Build history of the part. All positions in model axes, mm. A direction names the side the tool comes from. Give positions to 0.01 mm unless a question says otherwise; leave off trailing zeros. Loops run counter-clockwise (first coordinate to the right, second up) from the corner with the lowest first, then second, coordinate; pieces in that order, holes last. Notation, with made-up numbers: (44, -23.75) -> (75, -23.75) arc R15 ccw to (75, 0.25) -> close; hole circle Ø7 at (30, 8). An arc over 180 degrees is marked (long way). One line per question, with ' | ' between items. Start each with the question number.
(1) Slice it at C-C, the plane x = 30. Write the cut outline in (y, z).
(2) Drill centre lines: L1, parallel to X at y = 66.5, z = 31.5; L2, parallel to Y at x = 49, z = 38.5; L3, parallel to Z at x = 30, y = 0.8. Where is each one in solid material? Low to high. Write a range as from..to.
(3) Slice it at B-B, the plane z = 30. Write the cut outline in (x, y), then the cut area to 3 significant figures.
(4) Mould opens along X. For faces 1 (the face through (29.479, 1.014, 26.034)), 2 (the face through (108.99, 2.85, 29.58)), 3 (the face through (50, 0, 30)) say: pulls with the +X half, pulls with the -X half, needs draft (parallel to the pull), parting line crosses it, or undercut.
(5) 3-axis set-ups, long thin cutter, end or side, ignore diameter. For faces 4 (the face through (110, 64, 30)), 5 (the face through (110.986, 68.095, 29.133)): which of +Z, -Z, +X, -X, +Y, -Y reach the whole face in a straight line?
(6) Slice it at A-A, the plane y = 72. Write the cut outline in (x, z), then the cut area to 3 significant figures.
(7) Slice it at D-D, the plane z = 37. Write the cut outline in (x, y).
(8) Flat gauge pins, fed straight in: pin 1 Ø8 at (y, z) = (73.5, 32) entering from +X; pin 2 Ø18 at (y, z) = (61, 37) entering from -X; pin 3 Ø2 at (x, z) = (82, 43) entering from +Y; pin 4 Ø6.5 at (y, z) = (72, 30) entering from -X. Where does each tip first touch, or does it go through?
```python
from build123d import *

# Parameters (mm, degrees)
BOSS_EXTRUDE1_DEPTH = 60
SKETCH3_R           = 4
CUT_EXTRUDE1_DEPTH  = 3
SKETCH4_R           = 4
CUT_EXTRUDE2_DEPTH  = 3
FILLET3_R           = 10
FILLET4_R           = 10


with BuildPart() as part:
    # Sketch1 → Boss-Extrude1 (new body)
    with BuildSketch(Plane.XY):
        with BuildLine():
            Line((0, 0), (102, 0))
            ThreePointArc((102, 0), (109.071067812, 2.928932188), (112, 10))
            Line((112, 10), (112, 115))
            Line((112, 115), (110, 115))
            Line((110, 115), (110, 12))
            ThreePointArc((110, 12), (107.071067812, 4.928932188), (100, 2))
            Line((100, 2), (0, 2))
            Line((0, 2), (0, 0))
        make_face()
    extrude(amount=BOSS_EXTRUDE1_DEPTH)

    # Sketch3 → Cut-Extrude1 (cut, through all)
    with BuildSketch(Plane(origin=(0, 2, 0), x_dir=(1, 0, 0), z_dir=(0, 1, 0))):
        with Locations((30, -30)):
            Circle(SKETCH3_R)
    extrude(amount=-CUT_EXTRUDE1_DEPTH, mode=Mode.SUBTRACT)

    # Sketch4 → Cut-Extrude2 (cut, through all)
    with BuildSketch(Plane.ZY.offset(-110)):
        with Locations((30, 72)):
            Circle(SKETCH4_R)
    extrude(amount=-CUT_EXTRUDE2_DEPTH, mode=Mode.SUBTRACT)

    # Fillet3
    fillet3_edges = [part.edges().sort_by_distance(p)[0] for p in [
        (111, 115, 60),
        (111, 115, 0),
    ]]
    fillet(fillet3_edges, radius=FILLET3_R)

    # Fillet4
    fillet4_edges = [part.edges().sort_by_distance(p)[0] for p in [
        (0, 1, 0),
        (0, 1, 60),
    ]]
    fillet(fillet4_edges, radius=FILLET4_R)


solid = part.part
```
Final values:
1) outline: (0, 0) -> (2, 0) -> (2, 26) -> (0, 26) -> close; (0, 34) -> (2, 34) -> (2, 60) -> (0, 60) -> close
2) L1: 110..112 | L2: 0..2 | L3: 0..26, 34..60
3) outline: (0, 0) -> (26, 0) -> (26, 2) -> (0, 2) -> close; (34, 0) -> (102, 0) arc R10 ccw to (112, 10) -> (112, 68) -> (110, 68) -> (110, 12) arc R10 cw to (100, 2) -> (34, 2) -> close; (110, 76) -> (112, 76) -> (112, 115) -> (110, 115) -> close | area: 418 mm2
4) face 1: undercut | face 2: pulls with the +X half | face 3: needs draft
5) face 4: +Z, -Z, -X, +Y | face 5: +X, -X
6) outline: (110, 0) -> (112, 0) -> (112, 26) -> (110, 26) -> close; (110, 34) -> (112, 34) -> (112, 60) -> (110, 60) -> close | area: 104 mm2
7) outline: (0, 0) -> (102, 0) arc R10 ccw to (112, 10) -> (112, 115) -> (110, 115) -> (110, 12) arc R10 cw to (100, 2) -> (0, 2) -> close
8) pin 1: x = 112 | pin 2: x = 110 | pin 3: y = 2 | pin 4: through
